Geometry: final body of the model. Coordinates: model frame, mm. A direction names the side the tool comes from. Give positions to 0.01 mm unless a question says otherwise; leave off trailing zeros. Loops run counter-clockwise (first coordinate to the right, second up) from the corner with the lowest first, then second, coordinate; pieces in that order, holes last. Notation, with made-up numbers: (16.5, -18.5) -> (70.5, -18.5) arc R13 cw to (70.5, -0.5) -> close; hole circle Ø9 at (-3.5, 30.25). An arc over 180 degrees is marked (long way). Answer in a Markdown table with one row per item. Add a question column.
Autodesk Inventor part; units mm, degrees
ref_plane "YZ Plane" through (0, 0, 0) normal (1, 0, 0) x (0, 1, 0)
ref_plane "XZ Plane" through (0, 0, 0) normal (0, 1, 0) x (-1, 0, 0)
ref_plane "XY Plane" through (0, 0, 0) normal (0, 0, 1) x (1, 0, 0)
sketch "スケッチ1" plane through (0, 0, 0) normal (0, 0, 1) x (1, 0, 0)
  circle A0 centre (0, 0) radius 2
  circle A1 centre (15, 0) radius 2
  arc A2 (-0.2273, 4.9948) -> (-2.9263, -4.0542) centre (0, 0) ccw
  circle A3 centre (55, 0) radius 1.5
  circle A4 centre (55, 0) radius 4.025
  arc A5 (57.9262, 6.3865) -> (54.6807, 7.0177) centre (55, 0) ccw
  arc A6 (46.6204, -10.301) -> (48.0377, -5.2999) centre (45.4517, -7.2684) ccw
  line L0 (80, -19) -> (95, -19)
  circle A7 centre (95, -15) radius 2
  circle A8 centre (80, -15) radius 2
  arc A9 (95, -19) -> (96.6662, -11.3635) centre (95, -15) ccw
  circle A10 centre (80, -15) radius 4 construction
  line L1 (48.2385, -19) -> (80, -19)
  line L2 (57.9262, 6.3865) -> (96.6662, -11.3635)
  arc A11 (46.3293, 1.1755) -> (48.0377, -5.2999) centre (55, 0) ccw
  arc A12 (62.367, -1.4063) -> (54.6591, 7.4922) centre (55, 0) ccw
  line L3 (-0.2273, 4.9948) -> (54.6591, 7.4922)
  circle A13 centre (13, -10) radius 1.5
  arc A14 (10.3663, -13.6488) -> (12.3637, -14.4548) centre (13, -10) ccw
  line L4 (-2.9263, -4.0542) -> (10.3663, -13.6488)
  arc A15 (54.3637, -20.4538) -> (59.4202, -16.8428) centre (55, -15.999) ccw
  line L5 (12.3637, -14.4548) -> (54.3637, -20.4538)
  line L6 (59.4202, -16.8428) -> (62.367, -1.4063)
  circle A16 centre (66.7169, -2.5911) radius 1.5
  circle A17 centre (66.7169, -2.5911) radius 4.5 construction
  circle A18 centre (48.2385, -14.5) radius 1.5
  arc A19 (46.6204, -10.301) -> (48.2385, -19) centre (48.2385, -14.5) ccw
  arc A20 (80, -11) -> (80, -19) centre (80, -15) ccw
  line L7 (355.4948, -11) -> (390, -19)
  line L8 (390, -19) -> (80, -19)
  circle A21 centre (358.4948, -15) radius 1.25
  circle A22 centre (343.4948, -15) radius 1.25
  circle A23 centre (333.4948, -15) radius 1.25
  circle A24 centre (318.4948, -15) radius 1.25
  line L9 (80, -11) -> (207.8755, -11)
  line L10 (355.4948, -11) -> (248.9511, -11)
  arc A25 (213.7823, -10) -> (213.8378, -11) centre (210.8567, -10.6639) ccw
  line L11 (213.7823, -10) -> (214.7761, -9.8894)
  line L12 (213.8378, -11) -> (214.8378, -11)
  line L13 (219.357, -11) -> (218.357, -11)
  line L14 (218.2737, -9.5) -> (219.2676, -9.3894)
  line L15 (222.8762, -11) -> (223.8762, -11)
  line L16 (222.7652, -9) -> (223.7591, -8.8894)
  arc A26 (214.8378, -11) -> (218.357, -11) centre (216.5974, -10.3453) ccw
  arc A27 (218.2737, -9.5) -> (214.7761, -9.8894) centre (216.5974, -10.3453) ccw
  arc A28 (219.357, -11) -> (222.8762, -11) centre (221.1166, -10.0946) ccw
  arc A29 (222.7652, -9) -> (219.2676, -9.3894) centre (221.1166, -10.0946) ccw
  line L17 (210.8567, -10.6639) -> (233.0155, -9.4343) construction
  arc A30 (223.8762, -11) -> (229.892, -10.6107) centre (226.7628, -8.9308) ccw
  arc A31 (226.8407, -8.7739) -> (223.7591, -8.8894) centre (225.3075, -9.0352) ccw
  arc A32 (226.8407, -8.7739) -> (230.4998, -7.0068) centre (226.5478, -3.4953) ccw
  arc A33 (233.6316, -8.397) -> (230.4998, -7.0068) centre (231.2455, -9.5496) ccw
  arc A34 (235.4619, -12.6053) -> (229.892, -10.6107) centre (230.3136, -18.2076) ccw
  arc A35 (235.4619, -12.6053) -> (239.6511, -11) centre (234.0497, -2.6513) ccw
  arc A36 (259.6965, 4.4867) -> (265.8152, 14.9495) centre (248.2498, 18.2013) ccw
  arc A37 (220.191, -4.195) -> (265.8152, 14.9495) centre (219.3797, 61.6752) ccw
  line L18 (220.191, -4.195) -> (207.615, -4.3499)
  arc A38 (196.7777, -11) -> (207.615, -4.3499) centre (196.7777, 1.1554) ccw
  line L19 (222.8762, -11) -> (240.076, -10.0456) construction
  line L20 (222.7652, -9) -> (239.478, -8.0726) construction
  line L21 (239.6511, -11) -> (240.6511, -11)
  arc A39 (240.6511, -11) -> (242.7511, -11) centre (241.7011, -11) ccw
  line L22 (242.7511, -11) -> (243.7511, -11)
  arc A40 (243.7511, -11) -> (245.8511, -11) centre (244.8011, -11) ccw
  line L23 (245.8511, -11) -> (246.8511, -11)
  arc A41 (246.8511, -11) -> (248.9511, -11) centre (247.9011, -11) ccw
  arc A42 (240.735, -6.337) -> (238.7449, -7.0075) centre (239.7428, -6.6807) ccw
  arc A43 (243.5362, -5.2633) -> (241.5809, -6.0291) centre (242.5618, -5.6544) ccw
  arc A44 (246.2823, -4.0554) -> (244.3663, -4.9148) centre (245.3279, -4.4932) ccw
  arc A45 (248.9668, -2.7162) -> (247.0946, -3.6672) centre (248.0347, -3.1996) ccw
  arc A46 (233.6316, -8.397) -> (238.7449, -7.0075) centre (219.9279, 52.1342) ccw
  arc A47 (240.735, -6.337) -> (241.5809, -6.0291) centre (219.9279, 52.1342) ccw
  arc A48 (243.5362, -5.2633) -> (244.3663, -4.9148) centre (219.9279, 52.1342) ccw
  arc A49 (246.2823, -4.0554) -> (247.0946, -3.6672) centre (219.9279, 52.1342) ccw
  arc A50 (248.9668, -2.7162) -> (259.6965, 4.4867) centre (219.9279, 52.1342) ccw
  line L24 (196.7777, -11) -> (196.7777, -15)
  circle A51 centre (200.7777, -15) radius 1.25
  circle A52 centre (215.7777, -15) radius 1.25
  arc A53 (196.7777, -15) -> (200.7777, -19) centre (200.7777, -15) ccw
  arc A54 (215.7777, -19) -> (217.9536, -11.6436) centre (215.7777, -15) ccw
  circle A55 centre (200.7777, -15) radius 1.5
  circle A56 centre (215.7777, -15) radius 1.5
  line L25 (200.7777, -19) -> (215.7777, -19)
  circle A57 centre (45.4517, -7.2684) radius 1.5
  arc A58 (46.3293, 1.1755) -> (44.1782, 4.6812) centre (43.1088, 1.6121) ccw
  line L26 (54.6807, 7.0177) -> (44.8362, 6.5698)
  line L27 (44.8362, 6.5698) -> (44.1782, 4.6812)
  line L28 (355.4948, -11) -> (355.4948, -13)
  line L29 (355.4948, -13) -> (330.4948, -11)
  line L30 (330.4948, -11) -> (330.4948, -13)
  line L31 (330.4948, -13) -> (305.4948, -11)
  dimension "d0" = 4
  dimension "d1" = 4
  dimension "d2" = 15
  dimension "d3" = 3
  dimension "d4" = 3
  dimension "d8" = 8.05
  dimension "d9" = 3
  dimension "d10" = 6.5
  dimension "d11" = 4
  dimension "d12" = 4
  dimension "d15" = 15
  dimension "d16" = 15
  dimension "d18" = 3
  dimension "d19" = 3
  dimension "d23" = 3
  dimension "d25" = 40
  dimension "d26" = 40
  dimension "d28" = 15
  dimension "d29" = 13
  dimension "d34" = 3
  dimension "d35" = 3
  dimension "d36" = 3
  dimension "d37" = 8
  dimension "d38" = 390
  dimension "d40" = 4
  dimension "d41" = 8
  dimension "d42" = 2.5
  dimension "d43" = 2.5
  dimension "d44" = 2.5
  dimension "d45" = 2.5
  dimension "d46" = 4
  dimension "d47" = 15
  dimension "d48" = 10
  dimension "d49" = 15
  dimension "d51" = 6
  dimension "d59" = 1
  dimension "d60" = 1.5
  dimension "d61" = 1
  dimension "d62" = 1
  dimension "d63" = 1
  dimension "d64" = 2
  dimension "d65" = 1
  dimension "d66" = 1.0015
  dimension "d67" = 1.0015
  dimension "d68" = 0.7511
  dimension "d69" = 0.7511
  dimension "d70" = 3.176
  dimension "d71" = 3.176
  dimension "d73" = 1.05
  dimension "d74" = 1.05
  dimension "d75" = 1.05
  dimension "d76" = 1
  dimension "d77" = 1
  dimension "d78" = 1
  dimension "d79" = 2.1
  dimension "d80" = 2.1
  dimension "d81" = 2.1
  dimension "d82" = 2.1
  dimension "d83" = 3
  dimension "d84" = 3
  dimension "d85" = 3
  dimension "d88" = 2.5
  dimension "d89" = 2.5
  dimension "d90" = 15
extrude "押し出し1" add sketch "スケッチ1" along normal blind 6 contours L9 L24 A53 L8 A9 L2 | L2 A9 L0 A20 L9 | L9 A25 L12 A26 A54 L8 A53 L24 | A54 A26 L13 A28 L15 A30 A34 A35 L21 A39 L22 A40 L23 A41 L10 L31 L30 L29 L28 L7 L8 | A55 | A56
sketch "スケッチ2" plane through (0, 0, 6) normal (0, 0, 1) x (1, 0, 0)
  circle A0 centre (215.7777, -15) radius 1.25
  circle A1 centre (200.7777, -15) radius 1.25
  circle A2 centre (80, -15) radius 2
  circle A3 centre (95, -15) radius 2
  circle A4 centre (318.4948, -15) radius 1.25
  circle A5 centre (333.4948, -15) radius 1.25
  circle A6 centre (343.4948, -15) radius 1.25
  circle A7 centre (358.4948, -15) radius 1.25
  arc A8 (80, -11) -> (80, -19) centre (80, -15) ccw
  line L0 (80, -19) -> (390, -19)
  line L1 (390, -19) -> (355.4948, -11)
  line L2 (305.4948, -11) -> (248.9511, -11)
  arc A9 (246.8511, -11) -> (248.9511, -11) centre (247.9011, -11) ccw
  line L3 (246.8511, -11) -> (245.8511, -11)
  arc A10 (243.7511, -11) -> (245.8511, -11) centre (244.8011, -11) ccw
  line L4 (243.7511, -11) -> (242.7511, -11)
  arc A11 (240.6511, -11) -> (242.7511, -11) centre (241.7011, -11) ccw
  line L5 (240.6511, -11) -> (239.6511, -11)
  arc A12 (235.4619, -12.6053) -> (239.6511, -11) centre (234.0497, -2.6513) ccw
  arc A13 (235.4619, -12.6053) -> (229.892, -10.6107) centre (230.3136, -18.2076) ccw
  arc A14 (223.8762, -11) -> (229.892, -10.6107) centre (226.7628, -8.9308) ccw
  line L6 (223.8762, -11) -> (222.8762, -11)
  arc A15 (219.357, -11) -> (222.8762, -11) centre (221.1166, -10.0946) ccw
  line L7 (219.357, -11) -> (218.357, -11)
  arc A16 (214.8378, -11) -> (218.357, -11) centre (216.5974, -10.3453) ccw
  line L8 (214.8378, -11) -> (213.8378, -11)
  arc A17 (207.8755, -11) -> (213.8378, -11) centre (210.8567, -10.6639) ccw
  line L9 (207.8755, -11) -> (80, -11)
  circle A18 centre (105, -15) radius 2
  circle A19 centre (120, -15) radius 2
  arc A20 (105, -11) -> (105, -19) centre (105, -15) ccw
  line L10 (207.8755, -11) -> (80, -11)
  line L11 (330.4948, -11) -> (330.4948, -13)
  line L12 (330.4948, -13) -> (305.4948, -11)
  line L13 (355.4948, -11) -> (355.4948, -13)
  line L14 (355.4948, -13) -> (330.4948, -11)
  point P0 (0, 0)
  dimension "d114" = 4
  dimension "d115" = 4
  dimension "d116" = 15
  dimension "d117" = 4
  dimension "d119" = 25
extrude "押し出し2" cut sketch "スケッチ2" against normal blind 10 contours L9 A20 L0 A8 | A18 | A19
fillet "フィレット1" radius 0.5 1 edges at (390, -19, 3)
fillet "フィレット2" radius 1 2 edges at (355.4948, -13, 3) (330.4948, -13, 3)
sketch "スケッチ3" plane through (0, 0, 6) normal (0, 0, 1) x (1, 0, 0)
  arc A0 (385.6296, -19) -> (385.7426, -18.0129) centre (385.6296, -18.5) ccw
  line L0 (385.7426, -18.0129) -> (355.4948, -11)
  line L1 (355.4948, -11) -> (355.4948, -11.9168)
  arc A1 (354.4151, -12.9136) -> (355.4948, -11.9168) centre (354.4948, -11.9168) ccw
  line L2 (354.4151, -12.9136) -> (330.4948, -11)
  line L3 (330.4948, -11) -> (330.4948, -11.9168)
  arc A2 (329.4151, -12.9136) -> (330.4948, -11.9168) centre (329.4948, -11.9168) ccw
  line L4 (329.4151, -12.9136) -> (305.4948, -11)
  line L5 (305.4948, -11) -> (248.9511, -11)
  arc A3 (246.8511, -11) -> (248.9511, -11) centre (247.9011, -11) ccw
  line L6 (246.8511, -11) -> (245.8511, -11)
  arc A4 (243.7511, -11) -> (245.8511, -11) centre (244.8011, -11) ccw
  line L7 (243.7511, -11) -> (242.7511, -11)
  arc A5 (240.6511, -11) -> (242.7511, -11) centre (241.7011, -11) ccw
  line L8 (240.6511, -11) -> (239.6511, -11)
  arc A6 (235.4619, -12.6053) -> (239.6511, -11) centre (234.0497, -2.6513) ccw
  arc A7 (235.4619, -12.6053) -> (229.892, -10.6107) centre (230.3136, -18.2076) ccw
  arc A8 (223.8762, -11) -> (229.892, -10.6107) centre (226.7628, -8.9308) ccw
  line L9 (223.8762, -11) -> (222.8762, -11)
  arc A9 (219.357, -11) -> (222.8762, -11) centre (221.1166, -10.0946) ccw
  line L10 (219.357, -11) -> (218.357, -11)
  arc A10 (214.8378, -11) -> (218.357, -11) centre (216.5974, -10.3453) ccw
  line L11 (214.8378, -11) -> (213.8378, -11)
  arc A11 (207.8755, -11) -> (213.8378, -11) centre (210.8567, -10.6639) ccw
  line L12 (207.8755, -11) -> (105, -11)
  arc A12 (105, -11) -> (105, -19) centre (105, -15) ccw
  line L13 (105, -19) -> (385.6296, -19)
  circle A13 centre (318.4948, -15) radius 1.25
  circle A14 centre (333.4948, -15) radius 1.25
  circle A15 centre (343.4948, -15) radius 1.25
  circle A16 centre (358.4948, -15) radius 1.25
  circle A17 centre (200.7777, -15) radius 1.25
  circle A18 centre (215.7777, -15) radius 1.25
  circle A19 centre (120, -15) radius 2
  circle A20 centre (105, -15) radius 2
  line L14 (127, -15) -> (193.7777, -15) construction
  line L15 (127, -16.5) -> (193.7777, -16.5)
  line L16 (193.7777, -13.5) -> (127, -13.5)
  arc A21 (127, -13.5) -> (127, -16.5) centre (127, -15) ccw
  arc A22 (193.7777, -16.5) -> (193.7777, -13.5) centre (193.7777, -15) ccw
  line L17 (251.9511, -15) -> (305.4948, -15) construction
  line L18 (251.9511, -16.5) -> (305.4948, -16.5)
  line L19 (305.4948, -13.5) -> (251.9511, -13.5)
  arc A23 (251.9511, -13.5) -> (251.9511, -16.5) centre (251.9511, -15) ccw
  arc A24 (305.4948, -16.5) -> (305.4948, -13.5) centre (305.4948, -15) ccw
  point P0 (0, 0)
  point P1 (160.3889, -15)
  point P2 (278.723, -15)
  dimension "d129" = 3
  dimension "d130" = 3
  dimension "d131" = 7
  dimension "d132" = 7
  dimension "d133" = 3
  dimension "d134" = 0
extrude "押し出し3" cut sketch "スケッチ3" against normal blind 5 contours A21 L16 A22 L15 | A23 L19 A24 L18
properties part number "ロッド" material "アルミニウム 7075"
(1) Cut plane D-D on x = 323. Return the cut outline in (y, z).
(2) Draft query along Y for faces 4 (the flat face through (161, -13.5, 4)), 5 (the flat face through (318, -12, 3)), 6 (the flat face through (279, -13.5, 4)), 7 (the flat face through (242, -15, 0)). Return one class per face: +Y half, -Y half, draft (parallel to the pull), parting line (faces both ways), or undercut.
(3) Cut plane C-C on x = 204.5. Return the cut outline in (y, z), then the cut area to 3 significant figures.
(4) Pin query (flat end, axial travel): pin 1 Ø1.5 at (x, z) = (196, 1) entering from +Y; pin 2 Ø3.5 at (x, y) = (120, -15) entering from +Z. Return the tip coordinate at first contact, or that it passes through.
(5) Cut plane B-B on z = 4. State how many separate pieces and enclosed holes the cut face has, then the cut area to 3 significant figures.
(6) Reachability of faces 1 (the flat face through (343, -12, 3)), 2 (the flat face through (278, -11, 3)), 3 (the flat face through (278, -16.5, 4)) from +Z, -Z, +X, -X, +Y, -Y: full face, straight path, thin tool, end or side. Return the list, or none.
(7) Material intervals for line 1 along Y through (x, z) = (187.5, 1.1); line 2 along Y through (x, z) = (120, 1.2); line 3 along Y through (x, z) = (189, 0.75), sorted ascending. Write a range as from..to.
(8) Cut plane A-A on x = 262. Return the cut outline in (y, z), then the cut area to 3 significant figures.
Answer list:
| question | item | result |
|---|---|---|
| 1 | outline | (-19, 0) -> (-12.4, 0) -> (-12.4, 6) -> (-19, 6) -> close |
| 2 | face 4 | undercut |
| 2 | face 5 | +Y half |
| 2 | face 6 | undercut |
| 2 | face 7 | draft |
| 3 | outline | (-19, 0) -> (-11, 0) -> (-11, 6) -> (-19, 6) -> close |
| 3 | area | 48.0 mm² |
| 4 | pin 1 | stops at y = -11 |
| 4 | pin 2 | passes through |
| 5 | separate pieces | 1 |
| 5 | enclosed holes | 10 |
| 5 | area | 1,650 mm² |
| 6 | face 1 | +Z, -Z, +Y |
| 6 | face 2 | +Z, -Z, +X, +Y |
| 6 | face 3 | +Z |
| 7 | line 1 | y = -19..-16.5, -13.5..-11 |
| 7 | line 2 | y = -19..-17, -13..-11 |
| 7 | line 3 | y = -19..-11 |
| 8 | outline | (-19, 0) -> (-11, 0) -> (-11, 6) -> (-13.5, 6) -> (-13.5, 1) -> (-16.5, 1) -> (-16.5, 6) -> (-19, 6) -> close |
| 8 | area | 33.0 mm² |
